```python
from build123d import *


with BuildPart() as f1:
    # F0 (on Top) → F1 (revolve)
    with BuildSketch(Plane.XY):
        with BuildLine():
            Line((-3, 2.5), (-3, 1.5))
            Line((-3, 1.5), (3, 1.5))
            Line((3, 1.5), (3, 2.5))
            ThreePointArc((3, 2.5), (2.645751, 2.854249), (2.25, 3.161438))
            ThreePointArc((2.25, 3.161438), (0, 3.854249), (-2.25, 3.161438))
            ThreePointArc((-2.25, 3.161438), (-2.645751, 2.854249), (-3, 2.5))
        make_face()
        with BuildLine():
            Line((-2.25, 5.215143), (-2.25, 3.161438))
            ThreePointArc((-2.25, 3.161438), (0, 3.854249), (2.25, 3.161438))
            Line((2.25, 3.161438), (2.25, 5.215143))
            ThreePointArc((2.25, 5.215143), (0, 5.75), (-2.25, 5.215143))
        make_face()
    revolve(axis=Axis((0, 0, 0), (1, 0, 0)))

    # F2 (on Right) → F3 (revolve)
    with BuildSketch(Plane.YZ):
        Polygon((-12.5, 3.95), (-12.5, 0), (-3, 0), (-3, 3.5), (-7.5, 3.5), (-7.5, 4.45), (-8.5, 4.45), (-8.5, 3.95), align=None)
    revolve(axis=Axis((0, -6.25, 0), (0, -1, 0)))

    # F0 (on Top) → F4 (revolve, cut)
    with BuildSketch(Plane.XY):
        with BuildLine():
            Line((3, 2.5), (3, 1.5))
            Line((3, 1.5), (5, 1.5))
            Line((5, 1.5), (5, 6))
            Line((5, 6), (3.95, 6))
            Line((3.95, 6), (2.25, 5.215143))
            Line((2.25, 5.215143), (2.25, 3.161438))
            ThreePointArc((2.25, 3.161438), (2.645751, 2.854249), (3, 2.5))
        make_face()
        with BuildLine():
            Line((-5, 1.5), (-3, 1.5))
            Line((-3, 1.5), (-3, 2.5))
            ThreePointArc((-3, 2.5), (-2.645751, 2.854249), (-2.25, 3.161438))
            Line((-2.25, 3.161438), (-2.25, 5.215143))
            Line((-2.25, 5.215143), (-3.95, 6))
            Line((-3.95, 6), (-5, 6))
            Line((-5, 6), (-5, 1.5))
        make_face()
    revolve(axis=Axis((0, 0, 0), (1, 0, 0)), mode=Mode.SUBTRACT)


solid = f1.part
```
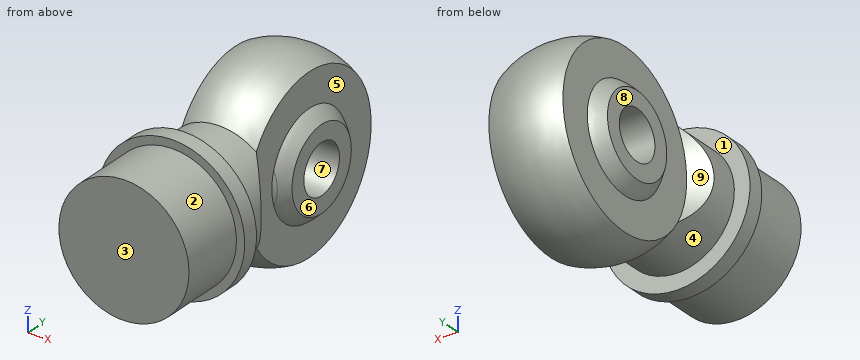
For this review, take the finished solid that the model builds, in its own axes (mm). Face numbers are marked on the shaded views. A direction names the side the tool comes from. Coordinates: 2 decimals unless noted, no trailing zeros. Write each loop counter-clockwise with the first axis right and the second up, starting at its lowest first coordinate (ties: lowest second). Pieces come first, ordered by that corner, then holes. Notation, with made-up numbers: (75, 11) - (86, 11) arc R20 cw to (86, 27) - close; hole circle Ø10 at (80.5, -35). An arc over 180 degrees is marked (long way). Put each result on its own line as item: value.
1. For pin 1 (6 mm diameter, centred on y = -3, z = -0.5, fed in from -X); pin 2 (1.5 mm diameter, centred on x = -0.5, z = 1, fed in from +Y); pin 3 (1.5 mm diameter, centred on y = 1, z = 0.5, fed in from -X), all flat-tipped, find the tip position at first contact; note any pin that passes through.
Values found:
pin 1: x = -3.5
pin 2: y = 5.74
pin 3: x = -3
2. Machinability: for the marked faces 5, 6, 7, 8 and 9, which of the approach directions +Z, -Z, +X, -X, +Y, -Y give a long, thin tool a straight path to every point of the face, cutting with its end or side? Answer none if there is none.
Values found:
face 5: +X
face 6: +Z, -Z, +X, +Y
face 7: +X, -X
face 8: +Z, -Z, -X, +Y
face 9: -X
3. Wall thickness on probe 1 along X at (y, z) = (-0.25, -3.25); probe 2 along X at (y, z) = (-6, -2.25); probe 3 along Z at (x, y) = (0.55, 0): over which ranges is each line inside the solid? List them lowest first.
Values found:
probe 1: -2.25 to 2.25
probe 2: -2.68 to 2.68
probe 3: -5.72 to -1.5, 1.5 to 5.72
4. Mouldability with a two-part tool opening along Y and no side actions: class the marked faces 1, 2, 3 and 4 as released by +Y, released by -Y, zero draft, split by the parting line, or undercut.
Values found:
face 1: undercut
face 2: zero draft
face 3: released by -Y
face 4: undercut
5. Add section B-B, the plane y = -10.25. Give the boundary of the cut face in (x, z), then the cut area to 3 significant figures.
Values found:
outline: circle Ø7.9 at (0, 0)
area: 49.0 mm²
6. Add section A-A, the plane y = -6.25. Give the boundary of the cut face in (x, z).
Values found:
outline: circle Ø7 at (0, 0)
